Model file for the job. Use its own axes, mm. A direction names the side the tool comes from. Coordinates: 2 decimals unless noted, no trailing zeros. Write each loop counter-clockwise with the first axis right and the second up, starting at its lowest first coordinate (ties: lowest second). Pieces come first, ordered by that corner, then holes.
Q1. Pull direction X, two halves, no side cores. Call faces 3 (the cylindrical face through (-46.105, 43.74, 0.035)), 4 (the flat face through (-41.805, 49, 0)), 5 (the flat face through (-64, 53.333, 0)), 6 (the flat face through (-7.77, 40.5, 0.04)): released by +X, released by -X, zero draft, split by the parting line, or undercut.
Q2. Band-saw the part on A-A, the plane x = -32.5. Write the cut outline in (y, z).
Q3. Band-saw the part on B-B, the plane y = 12. Write the cut outline in (x, z).
Q4. Which spindle directions (+Z, -Z, +X, -X, +Y, -Y) get a long thin tool onto all of the face, cutting with end or side? Do faces 1 (the cylindrical face through (7.46, 25.736, 0.035)), 2 (the flat face through (-60.605, 41, 0)). Say none if no direction does.
Q5. Drill centre lines: probe 1 along Y at (x, z) = (-41.5, 0.75); probe 2 along X at (y, z) = (39.2, 0); probe 3 along Y at (x, z) = (-52, 0). Where is each one in solid material? Low to high.
Q6. Pin check, flat tips, straight feed: P1, Ø1.2, axis at x = -58.5, z = -1.5, coming from the +Y side; P2, Ø2, axis at x = -59.21, z = 0, coming from the +Y side; P3, Ø2.5, axis at y = 50.5, z = 1, coming from the +X side. Stop position of each tip, or through.
from build123d import *

# Parameters (mm, degrees)
SKETCH_1_R          = 1.4
EXTRUDE_1_DEPTH     = 2.5
SKETCH_2_R          = 1.4
CUT_EXTRUDE_1_DEPTH = 0.1


with BuildPart() as part:
    # 草图1 → 凸台-拉伸1 (new body, symmetric)
    with BuildSketch(Plane.XY):
        with BuildLine():
            Line((-57.805032963, 53.332573096), (-44.605032963, 53.332573096))
            Line((-44.605032963, 53.332573096), (-44.605032963, 45.206973096))
            ThreePointArc((-44.605032963, 45.206973096), (-46.105032963, 43.706973096), (-44.605032963, 42.206973096))
            Line((-44.605032963, 42.206973096), (-44.605032963, 39.206973096))
            Line((-44.605032963, 39.206973096), (-41.805032963, 39.206973096))
            Line((-41.805032963, 39.206973096), (-41.805032963, 42.206973096))
            ThreePointArc((-41.805032963, 42.206973096), (-40.305032963, 43.706973096), (-41.805032963, 45.206973096))
            Line((-41.805032963, 45.206973096), (-41.805032963, 53.332573096))
            Line((-41.805032963, 53.332573096), (-28.605032963, 53.332573096))
            Line((-28.605032963, 53.332573096), (-28.605032963, 45.206973096))
            ThreePointArc((-28.605032963, 45.206973096), (-30.105032963, 43.706973096), (-28.605032963, 42.206973096))
            Line((-28.605032963, 42.206973096), (-28.605032963, 39.206973096))
            Line((-28.605032963, 39.206973096), (-25.805032963, 39.206973096))
            Line((-25.805032963, 39.206973096), (-25.805032963, 42.206973096))
            ThreePointArc((-25.805032963, 42.206973096), (-24.305032963, 43.706973096), (-25.805032963, 45.206973096))
            Line((-25.805032963, 45.206973096), (-25.805032963, 53.332573096))
            Line((-25.805032963, 53.332573096), (-20.605032963, 53.332573096))
            Line((-20.605032963, 53.332573096), (5.420799629, 27.306740503))
            ThreePointArc((5.420799629, 27.306740503), (7.491867441, 25.717554277), (9.90367699, 24.718550052))
            Line((9.90367699, 24.718550052), (81.270764772, 5.595796515))
            ThreePointArc((81.270764772, 5.595796515), (82.874367658, 4.524303323), (83.494307637, 2.698019036))
            Line((83.494307637, 2.698019036), (83.494307637, 0))
            Line((83.494307637, 0), (0, 0))
            Line((0, 0), (0, 7.857864376))
            ThreePointArc((0, 7.857864376), (-0.761204675, 11.6846987), (-2.928932188, 14.928932188))
            Line((-2.928932188, 14.928932188), (-19.524740269, 31.524740269))
            ThreePointArc((-19.524740269, 31.524740269), (-21.146857013, 32.608604026), (-23.060274175, 32.989206363))
            Line((-23.060274175, 32.989206363), (-62.648227072, 32.989206363))
            ThreePointArc((-62.648227072, 32.989206363), (-66.183760977, 34.453672457), (-67.648227072, 37.989206363))
            Line((-67.648227072, 37.989206363), (-67.648227072, 53.332573096))
            Line((-67.648227072, 53.332573096), (-60.605032963, 53.332573096))
            Line((-60.605032963, 53.332573096), (-60.605032963, 45.206973096))
            ThreePointArc((-60.605032963, 45.206973096), (-62.105032963, 43.706973096), (-60.605032963, 42.206973096))
            Line((-60.605032963, 42.206973096), (-60.605032963, 39.206973096))
            Line((-60.605032963, 39.206973096), (-57.805032963, 39.206973096))
            Line((-57.805032963, 39.206973096), (-57.805032963, 42.206973096))
            ThreePointArc((-57.805032963, 42.206973096), (-56.305032963, 43.706973096), (-57.805032963, 45.206973096))
            Line((-57.805032963, 45.206973096), (-57.805032963, 53.332573096))
        make_face()
        with Locations((45.49026085, 4.838412731)):
            Circle(SKETCH_1_R, mode=Mode.SUBTRACT)
        with Locations((61.49026085, 4.838412731)):
            Circle(SKETCH_1_R, mode=Mode.SUBTRACT)
    extrude(amount=EXTRUDE_1_DEPTH, both=True)

    # 草图2 → 切除-拉伸1 (cut)
    with BuildSketch(Plane(origin=(0, 39.206973096, 0), x_dir=(1, 0, 0), z_dir=(0, 1, 0))):
        with Locations((-59.205032963, 0)):
            Circle(SKETCH_2_R)
        with Locations((-43.205032963, 0)):
            Circle(SKETCH_2_R)
        with Locations((-27.205032963, 0)):
            Circle(SKETCH_2_R)
    extrude(amount=-CUT_EXTRUDE_1_DEPTH, mode=Mode.SUBTRACT)


solid = part.part
Answer sheet:
1. face 3: undercut
1. face 4: undercut
1. face 5: zero draft
1. face 6: released by +X
2. outline: (32.99, -2.5) - (53.33, -2.5) - (53.33, 2.5) - (32.99, 2.5) - close
3. outline: (-0.9, -2.5) - (57.37, -2.5) - (57.37, 2.5) - (-0.9, 2.5) - close
4. face 1: +Z, -Z, +X, +Y
4. face 2: +Z, -Z, +Y
5. probe 1: y = 32.99 to 42.24, 45.18 to 53.33
5. probe 2: x = -67.65 to -60.61, -57.81 to -44.61, -41.81 to -28.61, -25.81 to -6.47
5. probe 3: y = 32.99 to 53.33
6. P1: stops at y = 39.21
6. P2: stops at y = 39.11
6. P3: stops at x = -16.52
